```python
from build123d import *

# Parameters (mm, degrees)
SKETCH_W     = 42.3
SKETCH_H     = 42.3
SKETCH_R     = 1.8
SKETCH_R_2   = 11.5
PAD_DEPTH    = 52
SKETCH001_W  = 23
SKETCH001_H  = 30
POCKET_DEPTH = 21.15
CHAMFER_SIZE = 4
FILLET_R     = 2
FILLET001_R  = 2


with BuildPart() as part:
    # Sketch → Pad (new body)
    with BuildSketch(Plane.XY):
        with Locations((21.15, 21.15)):
            Rectangle(SKETCH_W, SKETCH_H)
        with Locations((5.65, 36.65)):
            Circle(SKETCH_R, mode=Mode.SUBTRACT)
        with Locations((36.65, 36.65)):
            Circle(SKETCH_R, mode=Mode.SUBTRACT)
        with Locations((36.65, 5.65)):
            Circle(SKETCH_R, mode=Mode.SUBTRACT)
        with Locations((5.65, 5.65)):
            Circle(SKETCH_R, mode=Mode.SUBTRACT)
        with Locations((21.15, 21.15)):
            Circle(SKETCH_R_2, mode=Mode.SUBTRACT)
    extrude(amount=PAD_DEPTH)

    # Sketch001 (on Face1 of Pad) → Pocket (cut)
    with BuildSketch(Plane(origin=(0, 42.3, 0), x_dir=(-1, 0, 0), z_dir=(0, 1, 0))):
        with Locations((-21.15, 21)):
            Rectangle(SKETCH001_W, SKETCH001_H)
    extrude(amount=-POCKET_DEPTH, mode=Mode.SUBTRACT)

    # Chamfer
    chamfer_edges = [part.edges().sort_by_distance(p)[0] for p in [
        (9.65, 42.3, 21),
        (32.65, 42.3, 21),
    ]]
    chamfer(chamfer_edges, length=CHAMFER_SIZE)

    # Fillet
    fillet_edges = [part.edges().sort_by_distance(p)[0] for p in [
        (42.3, 0, 26),
        (0, 0, 26),
        (42.3, 42.3, 26),
        (0, 42.3, 26),
    ]]
    fillet(fillet_edges, radius=FILLET_R)

    # Fillet001
    fillet001_edges = [part.edges().sort_by_distance(p)[0] for p in [
        (21.15, 42.3, 36),
        (21.15, 42.3, 6),
    ]]
    fillet(fillet001_edges, radius=FILLET001_R)


solid = part.part
```
The listing builds one solid part. Answer for the finished solid, in the listing's coordinates (mm). A direction names the side the tool comes from. Coordinates: 2 decimals unless noted, no trailing zeros. Loops run counter-clockwise (first coordinate to the right, second up) from the corner with the lowest first, then second, coordinate; pieces in that order, holes last. Notation, with made-up numbers: M 48,-37 L 103,-37 A10 cw 103,-26 Z; hole C 34,28.25 d3. An arc over 180 degrees is marked long. Answer as CSV lines item,"result". Start each with the question number.
(1) The part is cut by section A-A (y = 36.65). Give the vertices of the cut face in (x, z).
(2) Find the intervals of material crossed by L1, parallel to Y at x = 5.65, z = 20; L2, parallel to Z at x = 10, y = 31; L3, parallel to X at y = 21, z = 17, in increasing order. Write a range as [from, to].
(3) The part is cut by section D-D (x = 21.15). Give the vertices of the cut face in (y, z).
(4) The part is cut by section C-C (y = 5.65). Give the vertices of the cut face in (x, z).
(5) For faces 5 (the flat face through (34.62, 40.27, 20.76)), 6 (the flat face through (21, 42.3, 43)), determine the directions among +Z, -Z, +X, -X, +Y, -Y from which every point of the face is accessible in a straight line to the end or side of a thin tool.
(6) The mould has two halves that part along X. Classify faces 1 (the flat face through (9.65, 30, 21)), 2 (the cylindrical face through (41.7, 0.57, 26.36)), 3 (the flat face through (30, 12, 52)), 4 (the cylindrical face through (6.618, 7.168, 25.636)): pulls with the +X half, pulls with the -X half, needs draft (parallel to the pull), parting line crosses it, or undercut.
(7) The part is cut by section B-B (z = 47). Give the vertices of the cut face in (x, y), and give its area (3 significant figures).
Determined:
1,outline,"M 0,0 L 3.85,0 L 3.85,52 L 0,52 Z; M 7.45,0 L 34.85,0 L 34.85,52 L 7.45,52 Z; M 38.45,0 L 42.3,0 L 42.3,52 L 38.45,52 Z; hole M 9.65,6 L 32.65,6 L 32.65,36 L 9.65,36 Z"
2,L1,"[0, 3.85], [7.45, 34.85], [38.45, 42.3]"
2,L2,"[0, 6], [36, 52]"
2,L3,"[0, 9.65], [32.65, 42.3]"
3,outline,"M 0,0 L 9.65,0 L 9.65,52 L 0,52 Z; M 32.65,0 L 42.3,0 L 42.3,4 A2 ccw 40.3,6 L 32.65,6 Z; M 32.65,36 L 40.3,36 A2 ccw 42.3,38 L 42.3,52 L 32.65,52 Z"
4,outline,"M 0,0 L 3.85,0 L 3.85,52 L 0,52 Z; M 7.45,0 L 34.85,0 L 34.85,52 L 7.45,52 Z; M 38.45,0 L 42.3,0 L 42.3,52 L 38.45,52 Z"
5,face 5,"+Y"
5,face 6,"+Z, -Z, +X, -X, +Y"
6,face 1,"undercut"
6,face 2,"pulls with the +X half"
6,face 3,"needs draft"
6,face 4,"undercut"
7,outline,"M 0,2 A2 ccw 2,0 L 40.3,0 A2 ccw 42.3,2 L 42.3,40.3 A2 ccw 40.3,42.3 L 2,42.3 A2 ccw 0,40.3 Z; hole C 5.65,5.65 d3.6; hole C 5.65,36.65 d3.6; hole C 21.15,21.15 d23; hole C 36.65,5.65 d3.6; hole C 36.65,36.65 d3.6"
7,area,"1,330 mm2"
